from build123d import *

# Parameters (mm, degrees)
BOSS_EXTRUDE1_DEPTH = 6
M1_6_TAPPED_HOLE1_D = 1.25
SKETCH6_R           = 3.6
CUT_EXTRUDE1_DEPTH  = 20
SKETCH7_W           = 5.25
SKETCH7_H           = 7.2
CUT_EXTRUDE2_DEPTH  = 3


with BuildPart() as part:
    # Sketch1 → Boss-Extrude1 (new body)
    with BuildSketch(Plane(origin=(0, 0, 0), x_dir=(1, 0, 0), z_dir=(0, 1, 0))):
        Polygon((6, 2), (6, -13), (-4.5, -13), (-4.5, -2), (-4.5, 2), (1.5, 2), align=None)
    boss_extrude1 = extrude(amount=BOSS_EXTRUDE1_DEPTH)

    # Sketch3 → CSK SLOT for M1.6 Countersunk Flat Head Screw1 (revolve, cut)
    with BuildSketch(Plane(origin=(0.75, 6, 4.5), x_dir=(0, 0, 1), z_dir=(1, 0, 0))):
        Polygon((0, 0), (0, 6), (0.9, 6), (0.9, 4.9), (1.8, 4), (1.8, 0), align=None)
    csk_slot_for_m1_6_countersunk_flat_head = revolve(axis=Axis((0.75, 12.35, 4.5), (0, -1, 0)), mode=Mode.SUBTRACT)

    # M1.6 Tapped Hole1 (through all)
    with Locations(Plane(origin=(0, 6, 0), x_dir=(1, 0, 0), z_dir=(0, 1, 0))):
        with Locations((0.75, -9)):
            m1_6_tapped_hole1 = Hole(M1_6_TAPPED_HOLE1_D / 2)

    # Mirror1: Boss-Extrude1, CSK SLOT for M1.6 Countersunk Flat Head Screw1, M1.6 Tapped Hole1 across plane
    add(boss_extrude1.mirror(Plane(origin=(0, 0, -2), x_dir=(1, 0, 0), z_dir=(0, 0, -1))))
    add(csk_slot_for_m1_6_countersunk_flat_head.mirror(Plane(origin=(0, 0, -2), x_dir=(1, 0, 0), z_dir=(0, 0, -1))), mode=Mode.SUBTRACT)
    add(m1_6_tapped_hole1.mirror(Plane(origin=(0, 0, -2), x_dir=(1, 0, 0), z_dir=(0, 0, -1))), mode=Mode.SUBTRACT)

    # Sketch6 → Cut-Extrude1 (cut, through all)
    with BuildSketch(Plane(origin=(0, 6, 0), x_dir=(1, 0, 0), z_dir=(0, 1, 0))):
        with Locations(Location((0.75, 2, 0), (0, 0, 270))):
            Circle(SKETCH6_R)
    extrude(amount=-CUT_EXTRUDE1_DEPTH, mode=Mode.SUBTRACT)

    # Sketch7 → Cut-Extrude2 (cut)
    with BuildSketch(Plane(origin=(0, 6, 0), x_dir=(1, 0, 0), z_dir=(0, 1, 0))):
        with Locations((-1.875, 2)):
            Rectangle(SKETCH7_W, SKETCH7_H)
    extrude(amount=-CUT_EXTRUDE2_DEPTH, mode=Mode.SUBTRACT)


solid = part.part
Geometry: final body of the model. Coordinates: model frame, mm. A direction names the side the tool comes from. Round coordinates to 2 decimals unless told otherwise and drop trailing zeros. Loops run counter-clockwise (first coordinate to the right, second up) from the corner with the lowest first, then second, coordinate; pieces in that order, holes last. Notation, with made-up numbers: (-1, 13) -> (3, 13) arc R15 ccw to (3, 24) -> close; hole circle Ø11 at (35.5, 52). An arc over 180 degrees is marked (long way). One line per question, with ' | ' between items. Start each with the question number.
1. Section A-A on z = -2. Output: boundary loops of the cut face in (x, y), and give its area (4 significant figures).
2. Section C-C on y = 4.75. Output: boundary loops of the cut face in (x, z) (3 decimals).
3. Mould query, pull axis Z, two halves, no side actions, for faces 1 (the face through (0.7, 4, -6.7)), 2 (the face through (2, 0, 2)), 3 (the face through (1, 3, -17)), 4 (the face through (1, 3, 13)). Classes: pulls with the +Z half, pulls with the -Z half, needs draft (parallel to the pull), parting line crosses it, or undercut.
4. Contact query for flat-ended pins moving along their axis: pin 1 (2 mm diameter, centred on x = 0.75, z = -8.5, fed in from +Y); pin 2 (1 mm diameter, centred on x = 0.75, z = -13, fed in from +Y); pin 3 (2.5 mm diameter, centred on x = 0.75, z = 4.5, fed in from +Y). Output: stop coordinate, or through.
5. Section B-B on y = 0.4. Output: boundary loops of the cut face in (x, z) (3 decimals), and give its area (3 significant figures).
6. Line query: line 1 along Z through (x, y) = (0.75, 0.9) (3 decimals); line 2 along X through (y, z) = (4.2, 9) (3 decimals); line 3 along Z through (x, y) = (0.75, 4.8) (3 decimals). Output: solid intervals per line, ascending. Write a range as [from, to].
7. Set-up query: faces 5 (the face through (2, 6, 2)), 6 (the face through (-2, 5, 1.6)), 7 (the face through (1.439, 4.028, 6.163)). Return all of +Z, -Z, +X, -X, +Y, -Y with unobstructed straight access to the full face (end or side cutting, diameter ignored); none if empty.
8. Section D-D on z = 4.5. Output: boundary loops of the cut face in (x, y).
Returned:
1) outline: (-4.5, 0) -> (-2.85, 0) -> (-2.85, 3) -> (-4.5, 3) -> close; (4.35, 0) -> (6, 0) -> (6, 6) -> (4.35, 6) -> close | area: 14.85 mm2
2) outline: (-4.5, -17) -> (6, -17) -> (6, 13) -> (-4.5, 13) -> (-4.5, 1.6) -> (0.75, 1.6) arc R3.6 cw to (0.75, -5.6) -> (-4.5, -5.6) -> close; hole circle Ø3.6 at (0.75, -8.5); hole circle Ø3.6 at (0.75, 4.5); hole circle Ø1.25 at (0.75, -13); hole circle Ø1.25 at (0.75, 9)
3) face 1: undercut | face 2: needs draft | face 3: pulls with the -Z half | face 4: pulls with the +Z half
4) pin 1: stops at y = 1.2 | pin 2: passes through | pin 3: stops at y = 1.45
5) outline: (-4.5, -17) -> (6, -17) -> (6, 13) -> (-4.5, 13) -> close; hole circle Ø7.2 at (0.75, -2); hole circle Ø1.8 at (0.75, -8.5); hole circle Ø1.8 at (0.75, 4.5); hole circle Ø1.25 at (0.75, -13); hole circle Ø1.25 at (0.75, 9) | area: 267 mm2
6) line 1: z = [-17, -13.625], [-12.375, -9.4], [-7.6, -5.6], [1.6, 3.6], [5.4, 8.375], [9.625, 13] | line 2: x = [-4.5, 0.125], [1.375, 6] | line 3: z = [-17, -13.625], [-12.375, -10.3], [-6.7, -5.6], [1.6, 2.7], [6.3, 8.375], [9.625, 13]
7) face 5: +Z, -Z, +X, -X, +Y | face 6: -X, +Y | face 7: +Y
8) outline: (-4.5, 0) -> (-0.15, 0) -> (-0.15, 1.1) -> (-1.05, 2) -> (-1.05, 6) -> (-4.5, 6) -> close; (1.65, 0) -> (6, 0) -> (6, 6) -> (2.55, 6) -> (2.55, 2) -> (1.65, 1.1) -> close
